```python
from build123d import *

# Parameters (mm, degrees)
F0_R     = 45
F1_DEPTH = 20
F3_DEPTH = 18
F4_R     = 45
F5_DEPTH = 2


with BuildPart() as f1:
    # F0 (on Top) → F1 (new body)
    with BuildSketch(Plane.XY):
        Circle(F0_R)
    extrude(amount=F1_DEPTH)

    # F2 (on face) → F3 (cut)
    with BuildSketch(Plane.XY.offset(20)):
        with BuildLine():
            Line((29.241279, 14.899176), (32.773278, 1.717575))
            Line((32.773278, 1.717575), (44.938329, 2.355118))
            ThreePointArc((44.938329, 2.355118), (43.466662, 11.646857), (40.095294, 20.429572))
            Line((40.095294, 20.429572), (29.241279, 14.899176))
        make_face()
        with BuildLine():
            Line((27.523704, 17.874102), (37.740176, 24.508757))
            ThreePointArc((37.740176, 24.508757), (31.819805, 31.819805), (24.508757, 37.740176))
            Line((24.508757, 37.740176), (17.874102, 27.523704))
            Line((17.874102, 27.523704), (27.523704, 17.874102))
        make_face()
        with BuildLine():
            ThreePointArc((20.429572, 40.095294), (11.646857, 43.466662), (2.355118, 44.938329))
            Line((2.355118, 44.938329), (1.717575, 32.773278))
            Line((1.717575, 32.773278), (14.899176, 29.241279))
            Line((14.899176, 29.241279), (20.429572, 40.095294))
        make_face()
        with BuildLine():
            ThreePointArc((-40.095294, 20.429572), (-43.466662, 11.646857), (-44.938329, 2.355118))
            Line((-44.938329, 2.355118), (-32.773278, 1.717575))
            Line((-32.773278, 1.717575), (-29.241279, 14.899176))
            Line((-29.241279, 14.899176), (-40.095294, 20.429572))
        make_face()
        with BuildLine():
            ThreePointArc((-24.508757, 37.740176), (-31.819805, 31.819805), (-37.740176, 24.508757))
            Line((-37.740176, 24.508757), (-27.523704, 17.874102))
            Line((-27.523704, 17.874102), (-17.874102, 27.523704))
            Line((-17.874102, 27.523704), (-24.508757, 37.740176))
        make_face()
        with BuildLine():
            ThreePointArc((-2.355118, 44.938329), (-11.646857, 43.466662), (-20.429572, 40.095294))
            Line((-20.429572, 40.095294), (-14.899176, 29.241279))
            Line((-14.899176, 29.241279), (-1.717575, 32.773278))
            Line((-1.717575, 32.773278), (-2.355118, 44.938329))
        make_face()
        with BuildLine():
            ThreePointArc((-20.429572, -40.095294), (-11.646857, -43.466662), (-2.355118, -44.938329))
            Line((-2.355118, -44.938329), (-1.717575, -32.773278))
            Line((-1.717575, -32.773278), (-14.899176, -29.241279))
            Line((-14.899176, -29.241279), (-20.429572, -40.095294))
        make_face()
        with BuildLine():
            ThreePointArc((-37.740176, -24.508757), (-31.819805, -31.819805), (-24.508757, -37.740176))
            Line((-24.508757, -37.740176), (-17.874102, -27.523704))
            Line((-17.874102, -27.523704), (-27.523704, -17.874102))
            Line((-27.523704, -17.874102), (-37.740176, -24.508757))
        make_face()
        with BuildLine():
            ThreePointArc((-44.938329, -2.355118), (-43.466662, -11.646857), (-40.095294, -20.429572))
            Line((-40.095294, -20.429572), (-29.241279, -14.899176))
            Line((-29.241279, -14.899176), (-32.773278, -1.717575))
            Line((-32.773278, -1.717575), (-44.938329, -2.355118))
        make_face()
        with BuildLine():
            ThreePointArc((40.095294, -20.429572), (43.466662, -11.646857), (44.938329, -2.355118))
            Line((44.938329, -2.355118), (32.773278, -1.717575))
            Line((32.773278, -1.717575), (29.241279, -14.899176))
            Line((29.241279, -14.899176), (40.095294, -20.429572))
        make_face()
        with BuildLine():
            ThreePointArc((24.508757, -37.740176), (31.819805, -31.819805), (37.740176, -24.508757))
            Line((37.740176, -24.508757), (27.523704, -17.874102))
            Line((27.523704, -17.874102), (17.874102, -27.523704))
            Line((17.874102, -27.523704), (24.508757, -37.740176))
        make_face()
        with BuildLine():
            ThreePointArc((2.355118, -44.938329), (11.646857, -43.466662), (20.429572, -40.095294))
            Line((20.429572, -40.095294), (14.899176, -29.241279))
            Line((14.899176, -29.241279), (1.717575, -32.773278))
            Line((1.717575, -32.773278), (2.355118, -44.938329))
        make_face()
    extrude(amount=-F3_DEPTH, mode=Mode.SUBTRACT)

    # F4 (on face) → F5 (join)
    with BuildSketch(Plane.XY.offset(20)):
        Circle(F4_R)
    extrude(amount=F5_DEPTH)


solid = f1.part
```
Design review of the part built by this model. Coordinates are the model's own, in mm. A direction names the side the tool comes from. Round coordinates to 2 decimals unless told otherwise and drop trailing zeros. Write each loop counter-clockwise with the first axis right and the second up, starting at its lowest first coordinate (ties: lowest second). Pieces come first, ordered by that corner, then holes. Notation, with made-up numbers: (71.5, -36.75) -> (117.5, -36.75) arc R34 ccw to (117.5, 2.25) -> close; hole circle Ø11 at (21.5, 44.25). An arc over 180 degrees is marked (long way). Answer in a Markdown table with one row per item.
Q1. Take a section at A-A, the plane x = 23. State the section outline as (y, z) points.
The answers:
| item | result |
|---|---|
| outline | (-38.68, 0) -> (38.68, 0) -> (38.68, 22) -> (-38.68, 22) -> close; hole (-35.42, 2) -> (-22.4, 2) -> (-22.4, 20) -> (-35.42, 20) -> close; hole (22.4, 2) -> (35.42, 2) -> (35.42, 20) -> (22.4, 20) -> close |
Q2. Draft analysis for pull direction X (two halves, no side actions). For faces 1 (the face through (21.145, -32.56, 11.126)), 2 (the face through (20.765, -39.923, 10.846)), 3 (the face through (28, 28, 20)), state which applies: +X half, -X half, draft (parallel to the pull), parting line (faces both ways), or undercut.
The answers:
| item | result |
|---|---|
| face 1 | +X half |
| face 2 | parting line |
| face 3 | undercut |
Q3. Take a section at B-B, the plane y = 13. State the section outline as (x, z) points, then the cut area to 3 significant figures.
The answers:
| item | result |
|---|---|
| outline | (-43.08, 0) -> (43.08, 0) -> (43.08, 2) -> (29.75, 2) -> (29.75, 20) -> (43.08, 20) -> (43.08, 22) -> (-43.08, 22) -> (-43.08, 20) -> (-29.75, 20) -> (-29.75, 2) -> (-43.08, 2) -> close |
| area | 1,420 mm² |
Q4. Clearance check with flat-ended pins moving along their axes: pin 1 Ø5 at (x, z) = (-2.5, 11) entering from -Y; pin 2 Ø6 at (x, z) = (13.5, 3) entering from +Y; pin 3 Ø12 at (x, z) = (-10.5, 3) entering from +Y. State where each tip first meets the part, or that it passes through.
The answers:
| item | result |
|---|---|
| pin 1 | y = -45 |
| pin 2 | y = 43.72 |
| pin 3 | y = 44.77 |
Q5. To check wall thickness, follow L1, parallel to Z at x = -31, y = -28.5; L2, parallel to Y at x = -37.5, z = 9.75; L3, parallel to Y at x = -23, z = 4.25. State the ranges of each line that lie inside material, in increasing order. Write a range as [from, to].
The answers:
| item | result |
|---|---|
| L1 | [0, 2], [20, 22] |
| L2 | [-24.35, -19.11], [-1.97, 1.97], [19.11, 24.35] |
| L3 | [-38.68, -35.42], [-22.4, 22.4], [35.42, 38.68] |
Q6. Take a section at C-C, the plane x = -19. State the section outline as (y, z) points.
The answers:
| item | result |
|---|---|
| outline | (-40.79, 0) -> (40.79, 0) -> (40.79, 2) -> (37.29, 2) -> (37.29, 20) -> (40.79, 20) -> (40.79, 22) -> (-40.79, 22) -> (-40.79, 20) -> (-37.29, 20) -> (-37.29, 2) -> (-40.79, 2) -> close; hole (-29.26, 2) -> (-26.4, 2) -> (-26.4, 20) -> (-29.26, 20) -> close; hole (26.4, 2) -> (29.26, 2) -> (29.26, 20) -> (26.4, 20) -> close |
Q7. For faces 4 (the face through (-17.626, -34.592, 11.126)), 5 (the face through (2.04, 38.94, 11.13)), 6 (the face through (-21.238, -32.703, 11.126)), list the 3-axis set-ups (+Z, -Z, +X, -X, +Y, -Y) from which the entire face can be reached by the end or side of a thin tool; tool diameter is ignored.
The answers:
| item | result |
|---|---|
| face 4 | -Y |
| face 5 | none |
| face 6 | -X |
